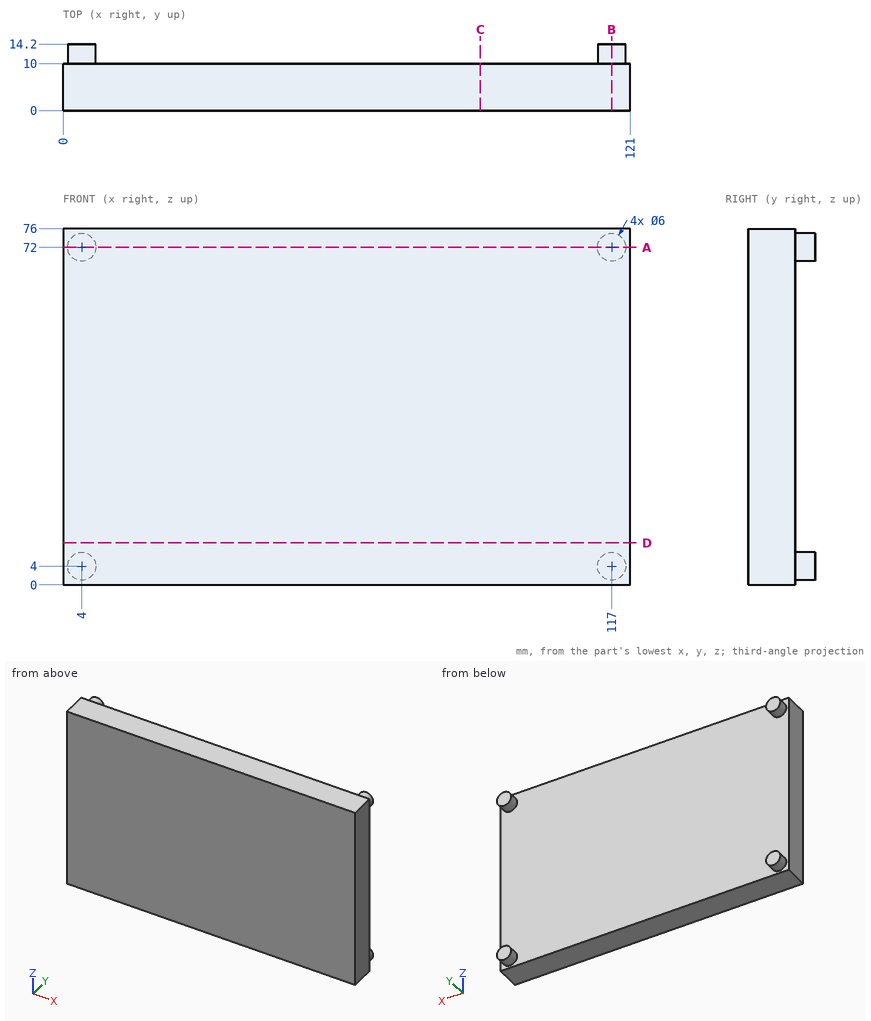
Part print with two shaded views. Sizes in mm from the minimum x, y, z corner. Coordinates: 2 decimals unless noted, no trailing zeros. Order: outer loops, then holes, each group sorted by start corner. A loop starts at its lowest first (then second) coordinate and runs counter-clockwise, first axis right, second up. Notation, with made-up numbers: M 32.25,86.5 L 89.25,86.5 A20 cw 89.25,102.5 Z; hole C 28,-34 d6. An arc over 180 degrees is marked long. Use a Markdown table: item, result.
(1) Cut at B-B on x = 117. Write the cut outline in (y, z).
A:
| item | result |
|---|---|
| outline | M 0,0 L 10,0 L 10,1 L 14.2,1 L 14.2,7 L 10,7 L 10,69 L 14.2,69 L 14.2,75 L 10,75 L 10,76 L 0,76 Z |
(2) Cut at A-A on z = 72. Write the cut outline in (x, y), then the cut area to 3 significant figures.
A:
| item | result |
|---|---|
| outline | M 0,0 L 121,0 L 121,10 L 120,10 L 120,14.2 L 114,14.2 L 114,10 L 7,10 L 7,14.2 L 1,14.2 L 1,10 L 0,10 Z |
| area | 1,260 mm^2 |
(3) Cut at C-C on x = 89. Write the cut outline in (y, z), then the cut area to 3 significant figures.
A:
| item | result |
|---|---|
| outline | M 0,0 L 10,0 L 10,76 L 0,76 Z |
| area | 760 mm^2 |
(4) Cut at D-D on z = 9. Write the cut outline in (x, y), then the cut area to 3 significant figures.
A:
| item | result |
|---|---|
| outline | M 0,0 L 121,0 L 121,10 L 0,10 Z |
| area | 1,210 mm^2 |
(5) Flat gauge pin, fed straight in: pin 1 (4 mm diameter, centred on x = 68.5, z = 60, fed in from +Y). Where does the tip first touch, or does it go through?
A:
| item | result |
|---|---|
| pin 1 | stops at y = 10 |
(6) Probe L1, parallel to X at y = 11.75, z = 4; L2, parallel to Y at x = 49.5, z = 49; L3, parallel to Z at x = 116, y = 13.25. List the from-to ranges inside material, lowest first.
A:
| item | result |
|---|---|
| L1 | x = 1 to 7, 114 to 120 |
| L2 | y = 0 to 10 |
| L3 | z = 1.17 to 6.83, 69.17 to 74.83 |
